Verification items for the finished model (mm, model axes). Round coordinates to 2 decimals unless told otherwise and drop trailing zeros. Write each loop counter-clockwise with the first axis right and the second up, starting at its lowest first coordinate (ties: lowest second). Pieces come first, ordered by that corner, then holes. Notation, with made-up numbers: M 35.5,23 L 57.5,23 A24 ccw 57.5,36 Z; hole C 5.25,53 d8. An arc over 180 degrees is marked long. One line per item, written item: value. Start each with the question number.
Item 1: Section check A-A, the plane y = 0. Record the cut outline in (x, z).
Item 2: Section check C-C, the plane z = 1.95. State how many separate pieces and enclosed holes the cut face has, then the cut area to 3 significant figures.
Item 3: Thickness scan on probe 1 along Y at (x, z) = (-15.5, 4.5); probe 2 along Y at (x, z) = (0, 2.55); probe 3 along Y at (x, z) = (6, 4.8). Record the ranges inside material, lowest first. Write a range as from..to.
Item 4: Gauge pin test, flat end, axial feed: pin 1 (10 mm diameter, centred on x = 3, y = -36.5, fed in from -Z). Record the tip position at first contact, or that the pin passes through.
Item 5: Draft check along X on faces 1 (the face through (42.9, 42.66, 2.54)), 2 (the face through (17.14, 20.12, 2.46)), 3 (the face through (35.99, 30.97, 2.46)), 4 (the face through (0, 47.173, 2)). Enter one of: +X half, -X half, draft (parallel to the pull), parting line (faces both ways), or undercut.
Item 6: Section check D-D, the plane x = -17. Record the cut outline in (y, z), then the cut area to 3 significant figures.
Autodesk Inventor part; units mm, degrees
ref_plane "YZ Plane" through (0, 0, 0) normal (1, 0, 0) x (0, 1, 0)
ref_plane "XZ Plane" through (0, 0, 0) normal (0, 1, 0) x (-1, 0, 0)
ref_plane "XY Plane" through (0, 0, 0) normal (0, 0, 1) x (1, 0, 0)
sketch "スケッチ1" plane through (0, 0, 0) normal (0, 0, 1) x (1, 0, 0)
  line L0 (-47.1734, 47.1734) -> (47.1734, 47.1734)
  line L1 (47.1734, 47.1734) -> (47.1734, -47.1734)
  line L2 (47.1734, -47.1734) -> (-47.1734, -47.1734)
  line L3 (-47.1734, -47.1734) -> (-47.1734, 47.1734)
  line L4 (-47.1734, 47.1734) -> (47.1734, -47.1734) construction
  line L5 (47.1734, 47.1734) -> (-47.1734, -47.1734) construction
  circle A0 centre (32.1734, 32.1734) radius 4
  circle A1 centre (-32.1734, 32.1734) radius 4
  circle A2 centre (-32.1734, -32.1734) radius 4
  circle A3 centre (32.1734, -32.1734) radius 4
  circle A4 centre (0, 0) radius 45.5 construction
  circle A5 centre (0, 0) radius 13.05
  circle A6 centre (0, 0) radius 25 construction
  circle A7 centre (17.6777, 17.6777) radius 2.5
  circle A8 centre (-17.6777, 17.6777) radius 2.5
  circle A9 centre (-17.6777, -17.6777) radius 2.5
  circle A10 centre (17.6777, -17.6777) radius 2.5
  line L6 (-7.8, -7.8) -> (7.8, 7.8) construction
  line L7 (7.8, -7.8) -> (-7.8, 7.8) construction
  line L8 (-17.6777, -17.6777) -> (-17.6777, 17.6777) construction
  line L9 (-17.6777, 17.6777) -> (17.6777, 17.6777) construction
  line L10 (17.6777, -17.6777) -> (-17.6777, -17.6777) construction
  line L11 (17.6777, -17.6777) -> (17.6777, 17.6777) construction
  dimension "d4" = 91
  dimension "d2" = 360
  dimension "d5" = 26.1
  dimension "d7" = 8
  dimension "d8" = 5
  dimension "d12" = 360
  dimension "d26" = 15
  dimension "d27" = 50
extrude "押し出し2" add sketch "スケッチ1" along normal blind 5
fillet "フィレット4" radius 15 4 edges at (47.1734, -47.1734, 2.5) (47.1734, 47.1734, 2.5) (-47.1734, -47.1734, 2.5) (-47.1734, 47.1734, 2.5)
properties part number "車輪ハブ1"
Response values:
1. outline: M -47.17,0 L -13.05,0 L -13.05,5 L -47.17,5 Z; M 13.05,0 L 47.17,0 L 47.17,5 L 13.05,5 Z
2. separate pieces: 1
2. enclosed holes: 9
2. area: 7,890 mm2
3. probe 1: y = -47.17..-18.91, -16.45..16.45, 18.91..47.17
3. probe 2: y = -47.17..-13.05, 13.05..47.17
3. probe 3: y = -47.17..-11.59, 11.59..47.17
4. pin 1: stops at z = 0
5. face 1: +X half
5. face 2: undercut
5. face 3: undercut
5. face 4: draft
6. outline: M -47.17,0 L -20.08,0 L -20.08,5 L -47.17,5 Z; M -15.27,0 L 15.27,0 L 15.27,5 L -15.27,5 Z; M 20.08,0 L 47.17,0 L 47.17,5 L 20.08,5 Z
6. area: 424 mm2
